The model under review builds one solid part; all positions refer to its coordinate system, in mm. Face numbers are marked on the shaded views. A direction names the side the tool comes from. Round coordinates to 2 decimals unless told otherwise and drop trailing zeros. Loops run counter-clockwise (first coordinate to the right, second up) from the corner with the lowest first, then second, coordinate; pieces in that order, holes last. Notation, with made-up numbers: M -21,73.5 L 6,73.5 A25 cw 6,106.5 Z; hole C 37.5,-3 d8. An arc over 180 degrees is marked long. Answer in a Markdown table with one row per item. Add a question column.
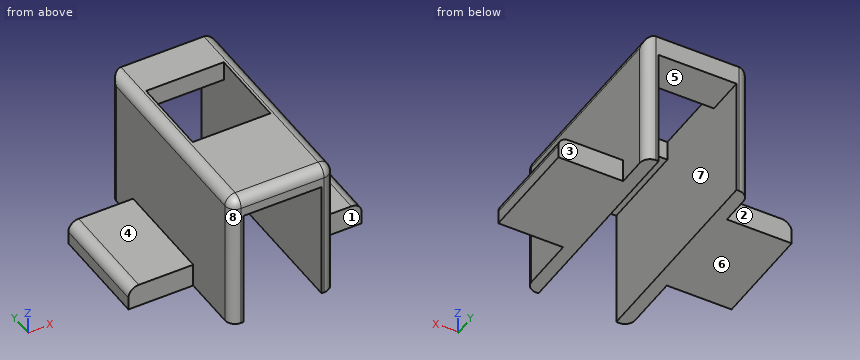
from build123d import *

# Parameters (mm, degrees)
F0_W     = 50.8
F0_H     = 101.6
F0_W_2   = 38.1
F0_H_2   = 12.7
F0_H_3   = 36.83
F1_DEPTH = 9.652
F2_W     = 50.8
F2_H     = 101.6
F3_DEPTH = 58.42
F4_W     = 31.75
F4_H     = 50.8
F5_DEPTH = 11.43
F6_R     = 5.08
F7_W     = 38.1
F7_H     = 58.42
F8_DEPTH = 101.601
F9_R     = 5.08


with BuildPart() as f1:
    # F0 (on Top) → F1 (new body)
    with BuildSketch(Plane.XY):
        with Locations((19.05, 44.45)):
            Rectangle(F0_W, F0_H)
        Polygon((38.1, 0), (0, 0), (0, 36.83), (0, 76.2), (0, 88.9), (38.1, 88.9), (38.1, 76.2), (38.1, 36.83), align=None, mode=Mode.SUBTRACT)
        with Locations((19.05, 82.55)):
            Rectangle(F0_W_2, F0_H_2)
        with Locations((19.05, 18.415)):
            Rectangle(F0_W_2, F0_H_3)
    extrude(amount=-F1_DEPTH)

    # F2 (on face) → F3 (join)
    with BuildSketch(Plane(origin=(0, 0, -9.652), x_dir=(1, 0, 0), z_dir=(0, 0, -1))):
        with Locations((19.05, -44.45)):
            Rectangle(F2_W, F2_H)
        Polygon((0, -36.83), (0, 0), (38.1, 0), (38.1, -36.83), (38.1, -76.2), (38.1, -88.9), (0, -88.9), (0, -76.2), align=None, mode=Mode.SUBTRACT)
    extrude(amount=F3_DEPTH)

    # F4 (on face) → F5 (join)
    with BuildSketch(Plane(origin=(0, 0, -68.072), x_dir=(1, 0, 0), z_dir=(0, 0, -1))):
        with Locations((60.325, -50.8)):
            Rectangle(F4_W, F4_H)
        with Locations((-22.225, -50.8)):
            Rectangle(F4_W, F4_H)
    extrude(amount=-F5_DEPTH)

    # F6
    f6_edges = [f1.edges().sort_by_distance(p)[0] for p in [
        (-38.1, 50.8, -56.642),
        (76.2, 50.8, -56.642),
    ]]
    fillet(f6_edges, radius=F6_R)

    # F7 (on face) → F8 (cut, through all)
    with BuildSketch(Plane.XZ.offset(6.35)):
        with Locations((19.05, -38.862)):
            Rectangle(F7_W, F7_H)
    extrude(amount=-F8_DEPTH, mode=Mode.SUBTRACT)

    # F9
    f9_edges = [f1.edges().sort_by_distance(p)[0] for p in [
        (19.05, -6.35, 0),
        (44.45, -6.35, -34.036),
        (-6.35, -6.35, -34.036),
        (44.45, 44.45, 0),
        (-6.35, 44.45, 0),
        (44.45, 95.25, -34.036),
        (-6.35, 95.25, -34.036),
    ]]
    fillet(f9_edges, radius=F9_R)


solid = f1.part
1. Mouldability with a two-part tool opening along X and no side actions: class the marked faces 6, 7 and 8 as released by +X, released by -X, zero draft, split by the parting line, or undercut.
2. Take a section at D-D, the plane z = -7. State the section outline as (x, y) points, and give its area (3 significant figures).
3. Take a section at A-A, the plane z = -44.5. State the section outline as (x, y) points, and give its area (3 significant figures).
4. Take a section at C-C, the plane y = 62.5. State the section outline as (x, z) points.
5. Take a section at B-B, the plane x = 20. State the section outline as (y, z) points, and give its area (3 significant figures).
6. For pin 1 Ø21 at (x, y) = (23.5, 82) entering from -Z; pin 2 Ø6 at (y, z) = (11.5, -46.5) entering from +X; pin 3 Ø5.5 at (x, z) = (-23, -63) entering from -Y, all flat-tipped, find the tip position at first contact; note any pin that passes through.
7. Machinability: for the marked faces 1, 2, 3, 4 and 5, which of the approach directions +Z, -Z, +X, -X, +Y, -Y give a long, thin tool a straight path to every point of the face, cutting with its end or side? Answer none if there is none.
8. To check wall thickness, follow probe 1 along X at (y, z) = (64, -15.5); probe 2 along Y at (x, z) = (1.5, -7). State the ranges of each line that lie inside material, in increasing order.
Check sheet entries:
| question | item | result |
|---|---|---|
| 1 | face 6 | zero draft |
| 1 | face 7 | undercut |
| 1 | face 8 | released by -X |
| 2 | outline | M -6.35,-1.27 A5.08 ccw -1.27,-6.35 L 39.37,-6.35 A5.08 ccw 44.45,-1.27 L 44.45,90.17 A5.08 ccw 39.37,95.25 L -1.27,95.25 A5.08 ccw -6.35,90.17 Z; hole M 0,36.83 L 38.1,36.83 L 38.1,76.2 L 0,76.2 Z |
| 2 | area | 3,640 mm^2 |
| 3 | outline | M -6.35,-1.27 A5.08 ccw -1.27,-6.35 L 0,-6.35 L 0,95.25 L -1.27,95.25 A5.08 ccw -6.35,90.17 Z; M 38.1,-6.35 L 39.37,-6.35 A5.08 ccw 44.45,-1.27 L 44.45,90.17 A5.08 ccw 39.37,95.25 L 38.1,95.25 Z |
| 3 | area | 1,270 mm^2 |
| 4 | outline | M -38.1,-68.07 L 0,-68.07 L 0,0 L -1.27,0 A5.08 ccw -6.35,-5.08 L -6.35,-56.64 L -33.02,-56.64 A5.08 ccw -38.1,-61.72 Z; M 38.1,-68.07 L 76.2,-68.07 L 76.2,-61.72 A5.08 ccw 71.12,-56.64 L 44.45,-56.64 L 44.45,-5.08 A5.08 ccw 39.37,0 L 38.1,0 Z |
| 5 | outline | M -6.35,-9.65 L 36.83,-9.65 L 36.83,0 L -1.27,0 A5.08 ccw -6.35,-5.08 Z; M 76.2,-9.65 L 95.25,-9.65 L 95.25,0 L 76.2,0 Z |
| 5 | area | 595 mm^2 |
| 6 | pin 1 | stops at z = -9.65 |
| 6 | pin 2 | stops at x = 44.45 |
| 6 | pin 3 | stops at y = 25.4 |
| 7 | face 1 | +Z, -Z, +X, -Y |
| 7 | face 2 | +Z, -Z, -X, +Y |
| 7 | face 3 | +Z, -Z, +X, +Y |
| 7 | face 4 | +Z, -X, +Y, -Y |
| 7 | face 5 | -Z, +Y, -Y |
| 8 | probe 1 | x = -6.35 to 0, 38.1 to 44.45 |
| 8 | probe 2 | y = -6.35 to 36.83, 76.2 to 95.25 |
